Model file for the job. Use its own axes, mm. Face numbers are marked on the shaded views. A direction names the side the tool comes from. Coordinates: 2 decimals unless noted, no trailing zeros. Order: outer loops, then holes, each group sorted by start corner. A loop starts at its lowest first (then second) coordinate and runs counter-clockwise, first axis right, second up. Notation, with made-up numbers: (-7.5, 18.5) -> (-2.5, 18.5) arc R17 cw to (-2.5, 48.5) -> close; hole circle Ø5 at (59.5, 27.25). An arc over 180 degrees is marked (long way). Return JSON: item names as keys, results as strings. Group by question number.
1) Which spindle directions (+Z, -Z, +X, -X, +Y, -Y) get a long thin tool onto all of the face, cutting with end or side? Do the marked faces 4, 5 and 6. Say none if no direction does.
2) Cut at A-A (y = 0). Write the cut outline in (x, z), and give its area (4 significant figures).
3) Flat gauge pins, fed straight in: pin 1 (3 mm diameter, centred on x = 2.5, z = 5.5, fed in from +Y); pin 2 (1.5 mm diameter, centred on x = -10.5, y = 6, fed in from -Z); pin 3 (17.5 mm diameter, centred on x = 2, y = 3.5, fed in from +Z); pin 4 (16 mm diameter, centred on x = 0, y = 0, fed in from +Z). Where does each tip first touch, or does it go through?
4) Probe line 1 (Y direction, x = 0, z = 3.9); line 2 (Y direction, x = 0, z = 0.8); line 3 (Z direction, x = -11, y = -8.5). List the from-to ranges inside material, lowest first.
5) Cut at D-D (y = -16). Write the cut outline in (x, z), and give its area (3 significant figures).
6) Pull direction X, two halves, no side cores. Call the marked faces 1, 2 and 3: +X half, -X half, draft (parallel to the pull), parting line (faces both ways), or undercut.
7) Cut at C-C (z = 2). Write the cut outline in (x, y), and give its area (3 significant figures).
Autodesk Inventor part; units mm, degrees
ref_plane "YZ Plane" through (0, 0, 0) normal (1, 0, 0) x (0, 1, 0)
ref_plane "XZ Plane" through (0, 0, 0) normal (0, 1, 0) x (-1, 0, 0)
ref_plane "XY Plane" through (0, 0, 0) normal (0, 0, 1) x (1, 0, 0)
sketch "Эскиз1" plane through (0, 0, 0) normal (0, 0, 1) x (1, 0, 0)
  line L0 (5.5, -5.5) -> (-5.5, -5.5)
  line L1 (-5.5, -5.5) -> (-5.5, 5.5)
  line L2 (-5.5, 5.5) -> (5.5, 5.5)
  line L3 (5.5, 5.5) -> (5.5, -5.5)
  line L4 (5.5, -5.5) -> (-5.5, 5.5) construction
  line L5 (-5.5, -5.5) -> (5.5, 5.5) construction
  circle A0 centre (0, 0) radius 20.45
  circle A1 centre (0, 0) radius 17.5
  dimension "d0" = 11
  dimension "d1" = 11
  dimension "d2" = 40.9
  dimension "d3" = 35
extrude "Выдавливание1" add sketch "Эскиз1" along normal blind 6 contours A0 | A1
sketch "Эскиз2" plane through (0, 0, 6) normal (0, 0, 1) x (1, 0, 0)
  circle A0 centre (0, 0) radius 19.5
  circle A1 centre (0, 0) radius 17.5
  dimension "d6" = 39
  dimension "d7" = 35
extrude "Выдавливание2" add sketch "Эскиз2" along normal blind 2
sketch "Эскиз3" plane through (0, 0, 0) normal (0, 0, -1) x (-1, 0, 0)
  circle A0 centre (0, 0) radius 16.95
  dimension "d10" = 33.9
extrude "Выдавливание3" cut sketch "Эскиз3" against normal blind 2.5
sketch "Эскиз4" plane through (0, 0, 6) normal (0, 0, 1) x (1, 0, 0)
  circle A0 centre (0, 0) radius 10
  dimension "d13" = 20
extrude "Выдавливание4" cut sketch "Эскиз4" against normal blind 10
properties part number "64t2018"
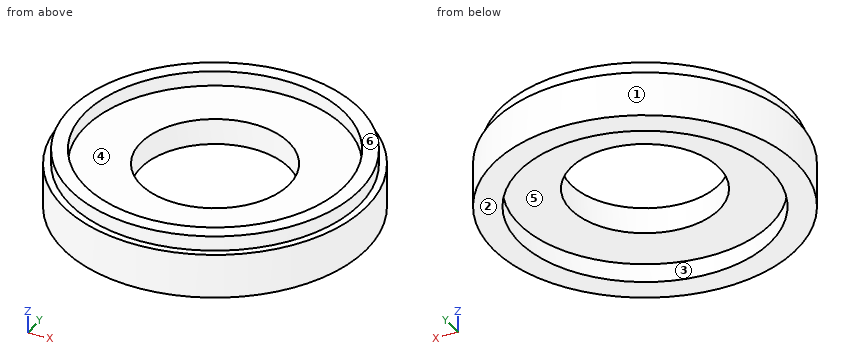
Answers below:
{
 "1": {"face 4": "+Z", "face 5": "-Z", "face 6": "+Z, +X, -X, +Y, -Y"},
 "2": {"outline": "(-20.45, 0) -> (-16.95, 0) -> (-16.95, 2.5) -> (-10, 2.5) -> (-10, 6) -> (-17.5, 6) -> (-17.5, 8) -> (-19.5, 8) -> (-19.5, 6) -> (-20.45, 6) -> close; (10, 2.5) -> (16.95, 2.5) -> (16.95, 0) -> (20.45, 0) -> (20.45, 6) -> (19.5, 6) -> (19.5, 8) -> (17.5, 8) -> (17.5, 6) -> (10, 6) -> close", "area": "98.65 mm^2"},
 "3": {"pin 1": "stops at y = 20.43", "pin 2": "stops at z = 2.5", "pin 3": "stops at z = 6", "pin 4": "passes through"},
 "4": {"line 1": "y = -20.45 to -10, 10 to 20.45", "line 2": "y = -20.45 to -16.95, 16.95 to 20.45", "line 3": "z = 2.5 to 6"},
 "5": {"outline": "(-12.74, 0) -> (-5.59, 0) -> (-5.59, 2.5) -> (5.59, 2.5) -> (5.59, 0) -> (12.74, 0) -> (12.74, 6) -> (11.15, 6) -> (11.15, 8) -> (7.09, 8) -> (7.09, 6) -> (-7.09, 6) -> (-7.09, 8) -> (-11.15, 8) -> (-11.15, 6) -> (-12.74, 6) -> close", "area": "141 mm^2"},
 "6": {"face 1": "parting line", "face 2": "draft", "face 3": "undercut"},
 "7": {"outline": "circle Ø40.9 at (0, 0); hole circle Ø33.9 at (0, 0)", "area": "411 mm^2"}
}
